Geometry check sheet. Reference: the model listing, model coordinates, mm. A direction names the side the tool comes from. Give positions to 0.01 mm unless a question says otherwise; leave off trailing zeros. Write each loop counter-clockwise with the first axis right and the second up, starting at its lowest first coordinate (ties: lowest second). Pieces come first, ordered by that corner, then holes. Notation, with made-up numbers: M 78,46 L 134,46 A13 ccw 134,57 Z; hole C 38.5,-28.5 d8. An arc over 180 degrees is marked long. One line per item, written item: value. Start each with the question number.
1. Scan lines: line 1 (Y direction, x = 0, z = 52.5); line 2 (Y direction, x = 0, z = 7.5); line 3 (X direction, y = -3, z = 51.5). Record each from-to range of solid material in increasing order.
2. Cross-section at D-D on z = 36. Record the cut outline in (x, y).
3. Release check for a two-part mould opening along Y. For faces 4 (the face through (0, 0, 47.625)), 5 (the face through (23.395, -7.367, 27.064)), 6 (the face through (4, 4, 57.15)) record: pulls with the +Y half, pulls with the -Y half, needs draft (parallel to the pull), parting line crosses it, or undercut.
4. Tool access check on faces 1 (the face through (-3.64, -27.7, 26.04)), 2 (the face through (-0.34, -1.55, 8.77)), 3 (the face through (-3.78, -2.9, 52.45)). Record the directions out of +Z, -Z, +X, -X, +Y, -Y that give a thin tool (end or side, any length) a straight path to the whole face; none if there is none.
5. Gauge pin test, flat ends, axial feed: pin 1 (5 mm diameter, centred on x = 22.5, z = 25.5, fed in from +Y); pin 2 (8 mm diameter, centred on x = 20.5, y = 5.5, fed in from -Z); pin 3 (8 mm diameter, centred on x = -18, y = -6.5, fed in from -Z). Record the tip position at first contact, or that the pin passes through.
6. Cross-section at C-C on z = 54.5. Record the cut outline in (x, y) (1 decimal), then the cut area to 3 significant figures.
from build123d import *

# Parameters (mm, degrees)
F2_R     = 1.5875
F4_DEPTH = 17.78
F3_R     = 4.7625
F5_DEPTH = 9.525


with BuildPart() as f1:
    # F0 (on Front) → F1 (revolve)
    with BuildSketch(Plane.XZ):
        with BuildLine():
            ThreePointArc((2.54, 0), (12.131985, 15.808015), (27.94, 25.4))
            Line((27.94, 25.4), (27.94, 26.67))
            Line((27.94, 26.67), (24.353637, 27.084503))
            ThreePointArc((24.353637, 27.084503), (19.770494, 30.074042), (15.726336, 33.760141))
            ThreePointArc((15.726336, 33.760141), (15.70698, 33.780889), (15.687641, 33.801654))
            ThreePointArc((15.687641, 33.801654), (11.774382, 38.898264), (8.89, 44.640161))
            Line((8.89, 44.640161), (8.89, 57.15))
            Line((8.89, 57.15), (0, 57.15))
            Line((0, 57.15), (0, 0))
            Line((0, 0), (2.54, 0))
        make_face()
    revolve(axis=Axis((0, 0, 28.575), (0, 0, -1)))

    # F2 (on Top) → F4 (cut)
    with BuildSketch(Plane.XY):
        Circle(F2_R)
    extrude(amount=F4_DEPTH, mode=Mode.SUBTRACT)

    # F3 (on face) → F5 (cut)
    with BuildSketch(Plane.XY.offset(57.15)):
        Circle(F3_R)
    extrude(amount=-F5_DEPTH, mode=Mode.SUBTRACT)


solid = f1.part
Report:
1. line 1: y = -8.89 to -4.76, 4.76 to 8.89
1. line 2: y = -5.81 to -1.59, 1.59 to 5.81
1. line 3: x = -8.37 to -3.7, 3.7 to 8.37
2. outline: C 0,0 d27.62
3. face 4: undercut
3. face 5: parting line crosses it
3. face 6: needs draft
4. face 1: +Z, -Z
4. face 2: -Z
4. face 3: +Z
5. pin 1: stops at y = 19.51
5. pin 2: stops at z = 20.1
5. pin 3: stops at z = 18.52
6. outline: C 0,0 d17.8; hole C 0,0 d9.5
6. area: 177 mm^2
